```python
from build123d import *

# Parameters (mm, degrees)
BOSS_EXTRUDE1_DEPTH = 5
SKETCH11_R          = 1.25
CUT_EXTRUDE1_DEPTH  = 31.149626863


with BuildPart() as part:
    # Sketch1 → Boss-Extrude1 (new body)
    with BuildSketch(Plane.XY):
        with BuildLine():
            Line((0, 20), (0, 10))
            Line((0, 10), (5, 10))
            ThreePointArc((5, 10), (11, 16), (17, 10))
            Line((17, 10), (22, 10))
            Line((22, 10), (22, 20))
            Line((22, 20), (0, 20))
        make_face()
        with BuildLine():
            Line((0, 10), (0, 0))
            Line((0, 0), (22, 0))
            Line((22, 0), (22, 10))
            Line((22, 10), (17, 10))
            ThreePointArc((17, 10), (11, 4), (5, 10))
            Line((5, 10), (0, 10))
        make_face()
    extrude(amount=BOSS_EXTRUDE1_DEPTH)

    # Sketch11 → Cut-Extrude1 (cut, through all)
    with BuildSketch(Plane(origin=(0, 20, 0), x_dir=(1, 0, 0), z_dir=(0, 1, 0))):
        with Locations(Location((2.25, -2.5, 0), (0, 0, 270))):
            Circle(SKETCH11_R)
        with Locations(Location((19.75, -2.5, 0), (0, 0, 90))):
            Circle(SKETCH11_R)
    extrude(amount=-CUT_EXTRUDE1_DEPTH, mode=Mode.SUBTRACT)


solid = part.part
```
Work out the finished part from the listing and answer in its coordinate system (mm). Round coordinates to 2 decimals unless told otherwise and drop trailing zeros. Loops run counter-clockwise (first coordinate to the right, second up) from the corner with the lowest first, then second, coordinate; pieces in that order, holes last. Notation, with made-up numbers: (23.25, 4) -> (39.25, 4) arc R31 ccw to (39.25, 38) -> close; hole circle Ø3 at (-36, 51). An arc over 180 degrees is marked (long way). Write each question's results on one line, items separated by ' | '. Start each with the question number.
1. For a pull along Z with two mould halves and no side action, classify faces 1 (the face through (11, 20, 2)), 2 (the face through (2.6, 10.1, 3.7)), 3 (the face through (16, 15, 0)) as +Z half, -Z half, draft (parallel to the pull), parting line (faces both ways), or undercut.
2. Section B-B (z = 2.5) is taken. Determine the outline of the cut face in (x, y).
3. Section D-D (y = 3.5) is taken. Determine the outline of the cut face in (x, z).
4. Section A-A (y = 10) is taken. Determine the outline of the cut face in (x, z).
5. Section C-C (x = 2.25) is taken. Determine the outline of the cut face in (y, z), plus the area to 3 significant figures.
6. Find the intervals of material crossed by probe 1 along X at (y, z) = (10.25, 2.5); probe 2 along Y at (x, z) = (11, 1.9); probe 3 along X at (y, z) = (13.75, 2.5), in increasing order. Write a range as from..to.
Evaluation:
1) face 1: draft | face 2: undercut | face 3: -Z half
2) outline: (0, 0) -> (1, 0) -> (1, 20) -> (0, 20) -> close; (3.5, 0) -> (18.5, 0) -> (18.5, 20) -> (3.5, 20) -> close; (21, 0) -> (22, 0) -> (22, 20) -> (21, 20) -> close; hole circle Ø12 at (11, 10)
3) outline: (0, 0) -> (22, 0) -> (22, 5) -> (0, 5) -> close; hole circle Ø2.5 at (2.25, 2.5); hole circle Ø2.5 at (19.75, 2.5)
4) outline: (0, 0) -> (5, 0) -> (5, 5) -> (0, 5) -> close; (17, 0) -> (22, 0) -> (22, 5) -> (17, 5) -> close; hole circle Ø2.5 at (2.25, 2.5); hole circle Ø2.5 at (19.75, 2.5)
5) outline: (0, 0) -> (20, 0) -> (20, 1.25) -> (0, 1.25) -> close; (0, 3.75) -> (20, 3.75) -> (20, 5) -> (0, 5) -> close | area: 50.0 mm2
6) probe 1: x = 0..1, 3.5..5.01, 16.99..18.5, 21..22 | probe 2: y = 0..4, 16..20 | probe 3: x = 0..1, 3.5..6.32, 15.68..18.5, 21..22
